Part model, mm, in its own coordinate system. A direction names the side the tool comes from. Round coordinates to 2 decimals unless told otherwise and drop trailing zeros. Loops run counter-clockwise (first coordinate to the right, second up) from the corner with the lowest first, then second, coordinate; pieces in that order, holes last. Notation, with made-up numbers: (-31.5, 45) - (-10.5, 45) arc R16 ccw to (-10.5, 69) - close; hole circle Ø6 at (22, -28). An arc over 180 degrees is marked (long way). Put each result on its own line as item: value.
from build123d import *

# Parameters (mm, degrees)
F0_R     = 11.15
F0_R_2   = 4
F1_DEPTH = 8
F0_R_3   = 7.15
F2_DEPTH = 1
F3_SIZE  = 0.5
F4_R     = 6
F4_R_2   = 4
F5_DEPTH = 1.5
F6_DEPTH = 20
F8_DEPTH = 25


with BuildPart() as f1:
    # F0 (on Top) → F1 (new body)
    with BuildSketch(Plane.XY):
        with BuildLine():
            ThreePointArc((14.310229, -52.917293), (91.75, 0), (14.310229, 52.917293))
            Line((14.310229, 52.917293), (-46.360014, 29.253574))
            ThreePointArc((-46.360014, 29.253574), (-66.35, 0), (-46.360014, -29.253574))
            Line((-46.360014, -29.253574), (14.310229, -52.917293))
        make_face()
        with BuildLine():
            Line((-44.543133, 24.595361), (16.12711, 48.25908))
            ThreePointArc((16.12711, 48.25908), (86.75, 0), (16.12711, -48.25908))
            Line((16.12711, -48.25908), (-44.543133, -24.595361))
            ThreePointArc((-44.543133, -24.595361), (-61.35, 0), (-44.543133, 24.595361))
        make_face(mode=Mode.SUBTRACT)
        with BuildLine():
            ThreePointArc((16.12711, -48.25908), (86.75, 0), (16.12711, 48.25908))
            Line((16.12711, 48.25908), (-44.543133, 24.595361))
            ThreePointArc((-44.543133, 24.595361), (-61.35, 0), (-44.543133, -24.595361))
            Line((-44.543133, -24.595361), (16.12711, -48.25908))
        make_face()
        with Locations((-34.95, 0)):
            Circle(F0_R, mode=Mode.SUBTRACT)
        with Locations((34.95, 0)):
            Circle(F0_R_2, mode=Mode.SUBTRACT)
    extrude(amount=F1_DEPTH)

    # F0 (on Top) → F2 (join)
    with BuildSketch(Plane.XY):
        with Locations((-34.95, 0)):
            Circle(F0_R)
        with Locations((-34.95, 0)):
            Circle(F0_R_3, mode=Mode.SUBTRACT)
    extrude(amount=F2_DEPTH)

    # F3
    f3_edges = [f1.edges().sort_by_distance(p)[0] for p in [
        (-46.1, 0, 8),
    ]]
    chamfer(f3_edges, length=F3_SIZE)

    # F4 (on face) → F5 (join)
    with BuildSketch(Plane.XY.offset(8)):
        with Locations((34.95, 0)):
            Circle(F4_R)
        with Locations((34.95, 0)):
            Circle(F4_R_2, mode=Mode.SUBTRACT)
    extrude(amount=F5_DEPTH)

    # F0 (on Top) → F6 (join)
    with BuildSketch(Plane.XY):
        with BuildLine():
            ThreePointArc((14.310229, -52.917293), (91.75, 0), (14.310229, 52.917293))
            Line((14.310229, 52.917293), (-46.360014, 29.253574))
            ThreePointArc((-46.360014, 29.253574), (-66.35, 0), (-46.360014, -29.253574))
            Line((-46.360014, -29.253574), (14.310229, -52.917293))
        make_face()
        with BuildLine():
            Line((-44.543133, 24.595361), (16.12711, 48.25908))
            ThreePointArc((16.12711, 48.25908), (86.75, 0), (16.12711, -48.25908))
            Line((16.12711, -48.25908), (-44.543133, -24.595361))
            ThreePointArc((-44.543133, -24.595361), (-61.35, 0), (-44.543133, 24.595361))
        make_face(mode=Mode.SUBTRACT)
    extrude(amount=F6_DEPTH)

    # F7 (on face) → F8 (cut)
    with BuildSketch(Plane.XY.offset(8)):
        with BuildLine():
            ThreePointArc((29.95, 41.49988), (24.774782, 40.542631), (19.760873, 38.942655))
            Line((19.760873, 38.942655), (-28.467059, 20.131915))
            ThreePointArc((-28.467059, 20.131915), (-19.459834, 14.400599), (-14.399513, 5))
            Line((-14.399513, 5), (19.751316, 5))
            ThreePointArc((19.751316, 5), (23.636292, 11.313708), (29.95, 15.198684))
            Line((29.95, 15.198684), (29.95, 41.49988))
        make_face()
        with BuildLine():
            ThreePointArc((76.44988, 5), (64.507063, 29.557063), (39.95, 41.49988))
            Line((39.95, 41.49988), (39.95, 15.198684))
            ThreePointArc((39.95, 15.198684), (46.263708, 11.313708), (50.148684, 5))
            Line((50.148684, 5), (76.44988, 5))
        make_face()
        with BuildLine():
            Line((19.751316, -5), (-14.399513, -5))
            ThreePointArc((-14.399513, -5), (-19.459834, -14.400599), (-28.467059, -20.131915))
            Line((-28.467059, -20.131915), (19.760873, -38.942655))
            ThreePointArc((19.760873, -38.942655), (24.774782, -40.542631), (29.95, -41.49988))
            Line((29.95, -41.49988), (29.95, -15.198684))
            ThreePointArc((29.95, -15.198684), (23.636292, -11.313708), (19.751316, -5))
        make_face()
        with BuildLine():
            ThreePointArc((39.95, -41.49988), (64.507063, -29.557063), (76.44988, -5))
            Line((76.44988, -5), (50.148684, -5))
            ThreePointArc((50.148684, -5), (46.263708, -11.313708), (39.95, -15.198684))
            Line((39.95, -15.198684), (39.95, -41.49988))
        make_face()
    extrude(amount=-F8_DEPTH, mode=Mode.SUBTRACT)


solid = f1.part
1. Band-saw the part on C-C (z = 15.25). List the corners of the cut face in (x, y), plus the area to 3 significant figures.
A:
outline: (-46.36, -29.25) - (14.31, -52.92) arc R56.8 ccw (long way) to (14.31, 52.92) - (-46.36, 29.25) arc R31.4 ccw to start; hole (-44.54, -24.6) - (16.13, -48.26) arc R51.8 ccw (long way) to (16.13, 48.26) - (-44.54, 24.6) arc R26.4 ccw to start
area: 2,050 mm²
2. Band-saw the part on D-D (z = 5.25). List the corners of the cut face in (x, y).
A:
outline: (-46.36, -29.25) - (14.31, -52.92) arc R56.8 ccw (long way) to (14.31, 52.92) - (-46.36, 29.25) arc R31.4 ccw to start; hole circle Ø22.3 at (-34.95, 0); hole (-28.47, -20.13) - (19.76, -38.94) arc R41.8 ccw to (29.95, -41.5) - (29.95, -15.2) arc R16 cw to (19.75, -5) - (-14.4, -5) arc R21.15 cw to start; hole (-28.47, 20.13) arc R21.15 cw to (-14.4, 5) - (19.75, 5) arc R16 cw to (29.95, 15.2) - (29.95, 41.5) arc R41.8 ccw to (19.76, 38.94) - close; hole circle Ø8 at (34.95, 0); hole (39.95, -41.5) arc R41.8 ccw to (76.45, -5) - (50.15, -5) arc R16 cw to (39.95, -15.2) - close; hole (39.95, 15.2) arc R16 cw to (50.15, 5) - (76.45, 5) arc R41.8 ccw to (39.95, 41.5) - close
3. Two-plate mould, pull along Y, no slides. Class faces 1 (the cylindrical face through (-19.36, -14.29, 4.06)), 2 (the cylindrical face through (-66.346, 0.527, 9.86)), 3 (the flat face through (6, 47, 20)): pulls with the +Y half, pulls with the -Y half, needs draft (parallel to the pull), parting line crosses it, or undercut.
A:
face 1: undercut
face 2: parting line crosses it
face 3: needs draft
4. Pin check, flat tips, straight feed: P1, Ø6, axis at y = 19, z = 8.5, coming from the +X side; P2, Ø9, axis at x = 1, z = 2, coming from the +Y side; P3, Ø8, axis at y = -7, z = 7.5, coming from the +X side; P4, Ø7, axis at x = 34.95, y = 0, coming from the -Z side. Stop position of each tip, or through.
A:
P1: stops at x = 89.45
P2: stops at y = 49.48
P3: stops at x = 91.67
P4: passes through
5. Probe line 1 along Y through (x, z) = (34.95, 7); line 2 along X through (y, z) = (-2, 7.5); line 3 along Y through (x, z) = (55, 6.25). List the from-to ranges inside material, lowest first. Write a range as [from, to].
A:
line 1: y = [-56.8, -4], [4, 56.8]
line 2: x = [-66.29, -45.92], [-23.98, 31.49], [38.41, 91.71]
line 3: y = [-53.14, -36.68], [-5, 5], [36.68, 53.14]
6. Band-saw the part on B-B (x = 34.95). List the corners of the cut face in (y, z).
A:
outline: (-56.8, 0) - (-4, 0) - (-4, 9.5) - (-6, 9.5) - (-6, 8) - (-51.8, 8) - (-51.8, 20) - (-56.8, 20) - close; (4, 0) - (56.8, 0) - (56.8, 20) - (51.8, 20) - (51.8, 8) - (6, 8) - (6, 9.5) - (4, 9.5) - close
7. Band-saw the part on A-A (y = 0). List the corners of the cut face in (x, z).
A:
outline: (-66.35, 0) - (-42.1, 0) - (-42.1, 1) - (-46.1, 1) - (-46.1, 7.5) - (-46.6, 8) - (-61.35, 8) - (-61.35, 20) - (-66.35, 20) - close; (-27.8, 0) - (30.95, 0) - (30.95, 9.5) - (28.95, 9.5) - (28.95, 8) - (-23.3, 8) - (-23.8, 7.5) - (-23.8, 1) - (-27.8, 1) - close; (38.95, 0) - (91.75, 0) - (91.75, 20) - (86.75, 20) - (86.75, 8) - (40.95, 8) - (40.95, 9.5) - (38.95, 9.5) - close
8. Tool access for faces 4 (the flat face through (63, 5, 4)), 5 (the flat face through (-35.1, -7.3, 1)): list every direction of +Z, -Z, +X, -X, +Y, -Y with a clear straight run to the whole face (end or side of a thin tool).
A:
face 4: +Z, -Z
face 5: +Z
